Part model, mm, in its own coordinate system. Face numbers are marked on the shaded views. Round coordinates to 2 decimals unless told otherwise and drop trailing zeros. Write each loop counter-clockwise with the first axis right and the second up, starting at its lowest first coordinate (ties: lowest second). Pieces come first, ordered by that corner, then holes.
1) Saw through at A-A on z = 26. Write the cut outline in (x, y), and give its area (3 significant figures).
2) Saw through at B-B on y = -6.5. Write the cut outline in (x, z), and give its area (3 significant figures).
3) Flat gauge pins, fed straight in: pin 1 (6 mm diameter, centred on x = 79, z = 33.5, fed in from -Y); pin 2 (6 mm diameter, centred on x = -28.5, y = -47.5, fed in from +Z); pin 3 (3 mm diameter, centred on x = 5.5, y = -36.5, fed in from -Z); pin 4 (5 mm diameter, centred on x = -13, y = -20, fed in from -Z). Where does each tip first touch, or does it go through?
4) Drill centre lines: L1, parallel to Y at x = 37, z = 18; L2, parallel to Z at x = 17, y = -18; L3, parallel to Y at x = 80, z = 0. Where is each one in solid material? Low to high.
5) Pull direction X, two halves, no side cores. Call the marked faces 1, 2 and 3: +X half, -X half, draft (parallel to the pull), parting line (faces both ways), or undercut.
```python
from build123d import *

# Parameters (mm, degrees)
F1_DEPTH = 112.7125
F2_R     = 6.35
F3_R     = 3.175
F5_DEPTH = 225.425


# Not quite as in the source:
# - a feature of the source that left no trace in its solid (it failed there, or was rolled back) is left out


with BuildPart() as f1:
    # F0 (on Right) → F1 (new body, symmetric)
    with BuildSketch(Plane.YZ):
        with BuildLine():
            ThreePointArc((-60.4918744543, 34.925), (-52.3875, 4.6790627728), (-30.2459372272, -17.4625))
            Line((-30.2459372272, -17.4625), (0, 0))
            Line((0, 0), (0, 34.925))
            ThreePointArc((0, 34.925), (-30.2459372272, 43.0293744543), (-60.4918744543, 34.925))
        make_face()
    extrude(amount=F1_DEPTH, both=True)

    # F2
    f2_edges = [f1.edges().sort_by_distance(p)[0] for p in [
        (0, -60.491874, 34.925),
        (0, 0, 0),
    ]]
    fillet(f2_edges, radius=F2_R)

    # F3
    f3_edges = [f1.edges().sort_by_distance(p)[0] for p in [
        (0, 0, 34.925),
        (0, -30.245937, -17.4625),
    ]]
    fillet(f3_edges, radius=F3_R)

    # F4 (on face) → F5 (cut, through all)
    with BuildSketch(Plane(origin=(-112.7125, 0, 0), x_dir=(0, -1, 0), z_dir=(-1, 0, 0))):
        Polygon((66.0401198141, 27.3149197272), (60.347308239, 30.7453752193), (31.890989487, -16.4776425833), (37.5838010621, -19.9080980754), align=None)
    extrude(amount=-F5_DEPTH, mode=Mode.SUBTRACT)


solid = f1.part
```
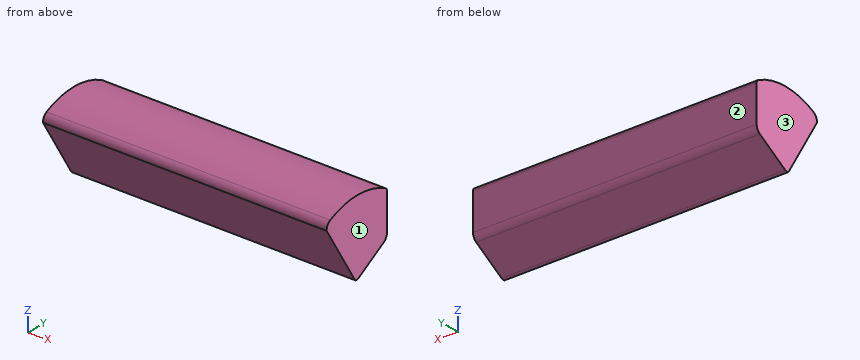
Completed:
1. outline: (-112.71, -57.49) - (112.71, -57.49) - (112.71, 0) - (-112.71, 0) - close
1. area: 13,000 mm2
2. outline: (-112.71, -3.75) - (112.71, -3.75) - (112.71, 38.17) - (-112.71, 38.17) - close
2. area: 9,450 mm2
3. pin 1: stops at y = -60.36
3. pin 2: stops at z = 41.33
3. pin 3: stops at z = -11.32
3. pin 4: stops at z = -12.99
4. L1: y = -52.67 to 0
4. L2: z = -10.39 to 41.78
4. L3: y = -41.82 to -1.17
5. face 1: +X half
5. face 2: draft
5. face 3: -X half
